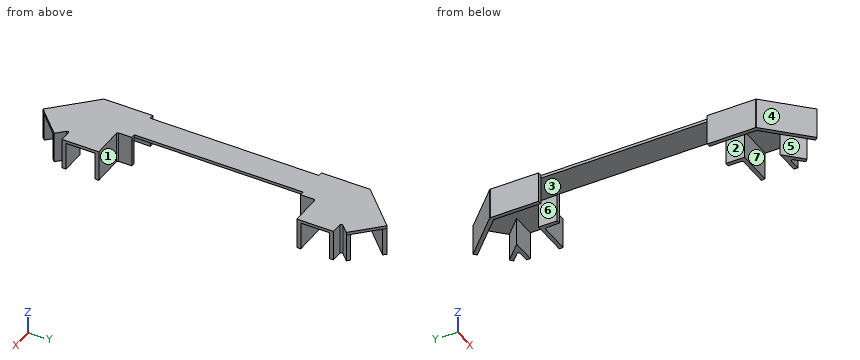
```python
from build123d import *

# Parameters (mm, degrees)
BOSS_EXTRUDE1_DEPTH = 2
SKETCH2_W           = 24.813601178
SKETCH2_H           = 2.7
BOSS_EXTRUDE2_DEPTH = 19
SKETCH3_W           = 25
SKETCH3_H           = 10
BOSS_EXTRUDE3_DEPTH = 2
SKETCH4_W           = 2.7
SKETCH4_H           = 10
BOSS_EXTRUDE4_DEPTH = 19
FILLET1_R           = 1


with BuildPart() as part:
    # Sketch1 → Boss-Extrude1 (new body)
    with BuildSketch(Plane.XY):
        Polygon((-9.5, -67.5), (-12.5, -67.5), (-12.5, -90.741737881), (14.006999461, -117.248737342), (31.68466899, -99.571067812), (24.613601178, -92.5), (34.613601178, -92.5), (34.613601178, -67.5), (9.5, -67.5), (9.5, 67.5), (34.613601178, 67.5), (34.613601178, 92.5), (24.613601178, 92.5), (31.68466899, 99.571067812), (14.006999461, 117.248737342), (-12.5, 90.741737881), (-12.5, 67.5), (-9.5, 67.5), align=None)
    extrude(amount=BOSS_EXTRUDE1_DEPTH)

    # Sketch2 → Boss-Extrude2 (add)
    with BuildSketch(Plane(origin=(0, 0, 0), x_dir=(-1, 0, 0), z_dir=(0, 0, -1))):
        Polygon((-34.613601178, 89.8), (-34.613601178, 92.5), (-24.613601178, 92.5), (-31.68466899, 99.571067812), (-29.775480681, 101.480256121), (-18.09522456, 89.8), align=None)
        with Locations((-22.206800589, 68.85)):
            Rectangle(SKETCH2_W, SKETCH2_H)
        Polygon((9.8, 67.5), (12.5, 67.5), (12.5, 90.741737881), (-14.006999461, 117.248737342), (-15.91618777, 115.339549032), (9.8, 89.623361262), align=None)
        Polygon((-31.68466899, -99.571067812), (-29.775480681, -101.480256121), (-18.09522456, -89.8), (-34.613601178, -89.8), (-34.613601178, -92.5), (-24.613601178, -92.5), align=None)
        with Locations((-22.206800589, -68.85)):
            Rectangle(SKETCH2_W, SKETCH2_H)
        Polygon((-14.006999461, -117.248737342), (-15.91618777, -115.339549032), (9.8, -89.623361262), (9.8, -67.5), (12.5, -67.5), (12.5, -90.741737881), align=None)
    extrude(amount=BOSS_EXTRUDE2_DEPTH)

    # Sketch3 → Boss-Extrude3 (add)
    with BuildSketch(Plane.XY.offset(2)):
        with Locations((0, -62.5)):
            Rectangle(SKETCH3_W, SKETCH3_H)
        with Locations((0, 62.5)):
            Rectangle(SKETCH3_W, SKETCH3_H)
    extrude(amount=-BOSS_EXTRUDE3_DEPTH)

    # Sketch4 → Boss-Extrude4 (add)
    with BuildSketch(Plane(origin=(0, 0, 0), x_dir=(-1, 0, 0), z_dir=(0, 0, -1))):
        with Locations((11.15, 62.5)):
            Rectangle(SKETCH4_W, SKETCH4_H)
        with Locations((-11.15, 62.5)):
            Rectangle(SKETCH4_W, SKETCH4_H)
        with Locations((11.15, -62.5)):
            Rectangle(SKETCH4_W, SKETCH4_H)
        with Locations((-11.15, -62.5)):
            Rectangle(SKETCH4_W, SKETCH4_H)
    extrude(amount=BOSS_EXTRUDE4_DEPTH)

    # Fillet1
    fillet1_edges = [part.edges().sort_by_distance(p)[0] for p in [
        (12.5, -67.5, -8.5),
        (12.5, 67.5, -8.5),
        (-12.5, 90.741737881, -8.5),
        (24.613601178, 92.5, -8.5),
        (24.613601178, -92.5, -8.5),
        (-12.5, -90.741737881, -8.5),
    ]]
    fillet(fillet1_edges, radius=FILLET1_R)


solid = part.part
```
Check sheet for the modelled part. Datum: model origin and axes. Units: mm. Face numbers are marked on the shaded views. A direction names the side the tool comes from. Coordinates: 2 decimals unless noted, no trailing zeros. Order: outer loops, then holes, each group sorted by start corner. A loop starts at its lowest first (then second) coordinate and runs counter-clockwise, first axis right, second up. Notation, with made-up numbers: (52.25, 78) -> (63.25, 78) arc R15 cw to (63.25, 107) -> close; hole circle Ø10 at (13, -31). An arc over 180 degrees is marked (long way). Write item = value, one per line. Start each with the question number.
1) Cross-section at C-C (z = -15). State how many separate pieces and enclosed holes the cut face has, then the cut area to 3 significant figures.
2) Go/stop test with flat-tipped pins: P1, Ø10, axis at y = 27, z = 0, coming from the +X side; P2, Ø9.5, axis at x = 21, z = -8, coming from the +Y side; P3, Ø7, axis at y = -62, z = -12, coming from the +X side; P4, Ø10, axis at x = 17, z = -16, coming from the +Y side. Record where each tip stops, or that it passes through.
3) Access from +Z, -Z, +X, -X, +Y, -Y to the whole of each face (thin tool, end or side, straight path). Record for the marked faces 5, 6 and 7.
4) Cross-section at A-A (x = 24). Enter the section's corners in (y, z), then the cut area to 3 significant figures.
5) Cross-section at B-B (y = 80.5). Enter the section's corners in (x, z), then the cut area to 3 significant figures.
6) Mould release check, pull along X, two halves, no side actions. Record for the marked faces 1, 2, 3 and 4: +X half, -X half, draft (parallel to the pull), parting line (faces both ways), or undercut.
7) Cross-section at D-D (x = -4.5). Enter the section's corners in (y, z), then the cut area to 3 significant figures.
8) Material ranges on L1, parallel to Y at x = 18, z = -8; L2, parallel to Y at x = 26.5, z = -0.25; L3, parallel to Y at x = 31, z = 1, recorded low to high.
Ans:
q1.separate_pieces = 6
q1.enclosed_holes = 0
q1.area = 710 mm²
q2.P1 = 9.5
q2.P2 = 97.45
q2.P3 = 12.5
q2.P4 = 117.25
q3.face_5 = -Z, -Y
q3.face_6 = -Z
q3.face_7 = -Z, +X
q4.outline = (-107.26, 0) -> (-95.7, 0) -> (-95.7, -19) -> (-89.8, -19) -> (-89.8, 0) -> (-70.2, 0) -> (-70.2, -19) -> (-67.5, -19) -> (-67.5, 2) -> (-107.26, 2) -> close; (67.5, -19) -> (70.2, -19) -> (70.2, 0) -> (89.8, 0) -> (89.8, -19) -> (95.7, -19) -> (95.7, 0) -> (107.26, 0) -> (107.26, 2) -> (67.5, 2) -> close
q4.area = 486 mm²
q5.outline = (-12.5, -19) -> (-9.8, -19) -> (-9.8, 0) -> (34.61, 0) -> (34.61, 2) -> (-12.5, 2) -> close
q5.area = 146 mm²
q6.face_1 = draft
q6.face_2 = undercut
q6.face_3 = undercut
q6.face_4 = -X half
q7.outline = (-98.74, -19) -> (-94.92, -19) -> (-94.92, 0) -> (94.92, 0) -> (94.92, -19) -> (98.74, -19) -> (98.74, 2) -> (-98.74, 2) -> close
q7.area = 540 mm²
q8.L1 = -70.2 to -67.5, 67.5 to 70.2
q8.L2 = -98.2 to -94.39, -92.65 to -89.8, -70.2 to -67.5, 67.5 to 70.2, 89.8 to 92.65, 94.39 to 98.2
q8.L3 = -100.26 to -98.89, -92.5 to -67.5, 67.5 to 92.5, 98.89 to 100.26
